For this review, take the finished solid that the model builds, in its own axes (mm). Face numbers are marked on the shaded views. A direction names the side the tool comes from. Coordinates: 2 decimals unless noted, no trailing zeros. Order: outer loops, then holes, each group sorted by start corner. A loop starts at its lowest first (then second) coordinate and runs counter-clockwise, first axis right, second up. Notation, with made-up numbers: (-35, 58) -> (-2, 58) arc R25 ccw to (-2, 76) -> close; hole circle Ø11 at (-8, 53). An arc over 180 degrees is marked (long way). Write item = value, one per line. Start each with the question number.
1) Consider section D-D on z = 9. Give the boundary of the cut face in (x, y), and give its area (3 significant figures).
2) Draft analysis for pull direction Z (two halves, no side actions). For the marked faces 1, 2, 3 and 4, state which applies: +Z half, -Z half, draft (parallel to the pull), parting line (faces both ways), or undercut.
3) Consider section A-A on x = 20. Give the boundary of the cut face in (y, z).
4) Insertion check: pin 1 Ø3 at (x, z) = (9.5, -10.5) entering from +Y; pin 2 Ø8 at (x, z) = (26, 9) entering from +Y; pin 3 Ø3 at (x, z) = (32.5, -8.5) entering from -Y. Each pin has a flat end and moves straight along its axis. Give the tip position at first contact, or say it passes through.
5) Wall thickness on probe 1 along Y at (x, z) = (19, 0); probe 2 along Y at (x, z) = (20, 3.5); probe 3 along Z at (x, y) = (35, -1.5): over which ranges is each line inside the solid? List them lowest first. Write a range as [from, to].
6) Consider section C-C on y = 1. Give the boundary of the cut face in (x, z), and give its area (3 significant figures).
7) Machinability: for the marked faces 5 and 6, which of the approach directions +Z, -Z, +X, -X, +Y, -Y give a long, thin tool a straight path to every point of the face, cutting with its end or side? Answer none if there is none.
from build123d import *

# Parameters (mm, degrees)
SKETCH1_R           = 6.4
BOSS_EXTRUDE1_DEPTH = 40
SKETCH3_R           = 6.4
CUT_EXTRUDE1_DEPTH  = 43


with BuildPart() as part:
    # Sketch1 → Boss-Extrude1 (new body)
    with BuildSketch(Plane(origin=(0, 0, 0), x_dir=(0, 0, -1), z_dir=(1, 0, 0))):
        with BuildLine():
            Line((15, 0), (15, 35))
            Line((15, 35), (-15, 35))
            Line((-15, 35), (-15, 0))
            ThreePointArc((-15, 0), (0, -15), (15, 0))
        make_face()
        Circle(SKETCH1_R, mode=Mode.SUBTRACT)
    extrude(amount=BOSS_EXTRUDE1_DEPTH)

    # Sketch3 → Cut-Extrude1 (cut)
    with BuildSketch(Plane(origin=(0, 0, -15), x_dir=(-1, 0, 0), z_dir=(0, 0, -1))):
        with Locations((-20, 20)):
            Circle(SKETCH3_R)
        with BuildLine():
            Line((-46.007478206, 15), (-34.81696458, 15))
            Line((-34.81696458, 15), (-34.877252069, 19.610892924))
            ThreePointArc((-34.877252069, 19.610892924), (-20.194570167, 34.8810677), (-5.11766035, 20))
            Line((-5.11766035, 20), (-5.11766035, 15))
            Line((-5.11766035, 15), (8.555205081, 15))
            Line((8.555205081, 15), (8.555205081, 43.038004213))
            Line((8.555205081, 43.038004213), (-46.007478206, 43.038004213))
            Line((-46.007478206, 43.038004213), (-46.007478206, 15))
        make_face()
    extrude(amount=-CUT_EXTRUDE1_DEPTH, mode=Mode.SUBTRACT)


solid = part.part
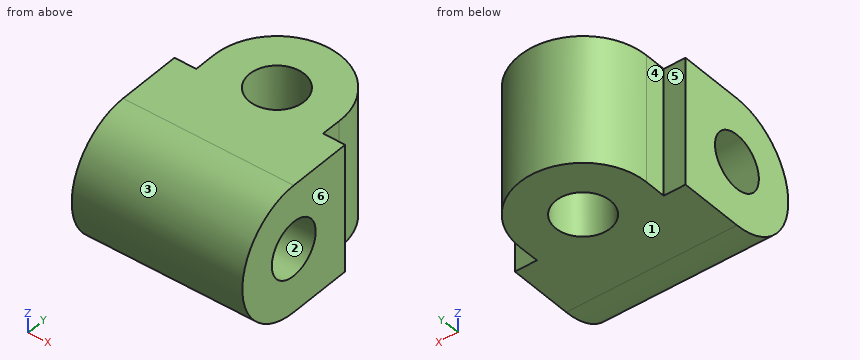
Answer sheet:
q1.outline = (0, -12) -> (40, -12) -> (40, 15) -> (34.82, 15) -> (34.88, 19.61) arc R14.88 ccw (long way) to (5.12, 20) -> (5.12, 15) -> (0, 15) -> close; hole circle Ø12.8 at (20, 20)
q1.area = 1,450 mm2
q2.face_1 = -Z half
q2.face_2 = undercut
q2.face_3 = parting line
q2.face_4 = draft
q3.outline = (0, -15) -> (13.6, -15) -> (13.6, 15) -> (0, 15) arc R15 ccw to start; (26.4, -15) -> (34.88, -15) -> (34.88, 15) -> (26.4, 15) -> close; hole circle Ø12.8 at (0, 0)
q4.pin_1 = 31.85
q4.pin_2 = 34.75
q4.pin_3 = -13.27
q5.probe_1 = [-15, -6.4], [6.4, 13.68], [26.32, 34.85]
q5.probe_2 = [-14.59, -5.36], [5.36, 13.6], [26.4, 34.88]
q5.probe_3 = [-14.92, -6.22], [6.22, 14.92]
q6.outline = (0, -15) -> (40, -15) -> (40, -6.32) -> (0, -6.32) -> close; (0, 6.32) -> (40, 6.32) -> (40, 15) -> (0, 15) -> close
q6.area = 694 mm2
q7.face_5 = +Z, -Z, -X, +Y
q7.face_6 = +Z, -Z, +X, +Y, -Y
